from build123d import *

# Parameters (mm, degrees)
EXTRUDE_1_DEPTH     = 6.25
SKETCH_2_R          = 4
CUT_EXTRUDE_1_DEPTH = 20
SKETCH_3_R          = 4
CUT_EXTRUDE_2_DEPTH = 62.216827752
SKETCH_4_W          = 7
SKETCH_4_H          = 36
CUT_EXTRUDE_3_DEPTH = 62.216827752


with BuildPart() as part:
    # Эскиз1 → Бобышка-Вытянуть1 (new, symmetric)
    with BuildSketch(Plane(origin=(0, 0, 0), x_dir=(0, 0, -1), z_dir=(1, 0, 0))):
        Polygon((0, 49), (0, -49), (-12, -49), (-34.5, -43), (-34.5, 43), (-12, 49), align=None)
    extrude(amount=EXTRUDE_1_DEPTH, both=True)

    # Эскиз2 → Вырез-Вытянуть1 (cut)
    with BuildSketch(Plane.XY.offset(34.5)):
        with Locations((0, -5)):
            Circle(SKETCH_2_R)
        with Locations((0, -15)):
            Circle(SKETCH_2_R)
        with Locations((0, -25)):
            Circle(SKETCH_2_R)
        with Locations(Location((0, 25, 0), (0, 0, 180))):
            Circle(SKETCH_2_R)
        with Locations(Location((0, 15, 0), (0, 0, 180))):
            Circle(SKETCH_2_R)
        with Locations(Location((0, 5, 0), (0, 0, 180))):
            Circle(SKETCH_2_R)
        with Locations((0, -35)):
            Circle(SKETCH_2_R)
        with Locations(Location((0, 35, 0), (0, 0, 180))):
            Circle(SKETCH_2_R)
    extrude(amount=-CUT_EXTRUDE_1_DEPTH, mode=Mode.SUBTRACT)

    # Эскиз3 → Вырез-Вытянуть2 (cut, through all)
    with BuildSketch(Plane(origin=(6.25, 0, 0), x_dir=(0, 0, -1), z_dir=(1, 0, 0))):
        with Locations((-24.5, -35)):
            Circle(SKETCH_3_R)
        with Locations((-24.5, -25)):
            Circle(SKETCH_3_R)
        with Locations((-24.5, -15)):
            Circle(SKETCH_3_R)
        with Locations((-24.5, -5)):
            Circle(SKETCH_3_R)
        with Locations((-24.5, 5)):
            Circle(SKETCH_3_R)
        with Locations((-24.5, 15)):
            Circle(SKETCH_3_R)
        with Locations((-24.5, 25)):
            Circle(SKETCH_3_R)
        with Locations((-24.5, 35)):
            Circle(SKETCH_3_R)
    extrude(amount=-CUT_EXTRUDE_2_DEPTH, mode=Mode.SUBTRACT)

    # Эскиз4 → Вырез-Вытянуть3 (cut, through all)
    with BuildSketch(Plane.ZY.offset(6.25)):
        with Locations((3.5, 0)):
            Rectangle(SKETCH_4_W, SKETCH_4_H)
    extrude(amount=-CUT_EXTRUDE_3_DEPTH, mode=Mode.SUBTRACT)


solid = part.part
Design review of the part built by this model. Coordinates are the model's own, in mm. A direction names the side the tool comes from. Give positions to 0.01 mm unless a question says otherwise; leave off trailing zeros. Loops run counter-clockwise (first coordinate to the right, second up) from the corner with the lowest first, then second, coordinate; pieces in that order, holes last. Notation, with made-up numbers: M 62.5,63 L 90.5,63 A8 cw 90.5,70 Z; hole C 43,48 d5. An arc over 180 degrees is marked long. One line per question, with ' | ' between items. Start each with the question number.
1. To check wall thickness, follow L1, parallel to X at y = -25, z = 19.25; L2, parallel to Y at x = 2.5, z = 6; L3, parallel to Z at x = -4.25, y = 15. State the ranges of each line that lie inside material, in increasing order.
2. The part is to be moulded in two halves that separate along Z. For faces 1 (the face through (0, -49, 6)), 2 (the face through (-4.47, -1.034, 25.021)), 3 (the face through (0, -33, 0)), say which applies: released by +Z, released by -Z, zero draft, split by the parting line, or undercut.
3. Add section B-B (z = 18.5). Give the number of separate pieces and of enclosed holes in the cut face, plus the area to 3 significant figures.
4. Add section A-A (y = -35). Write out the cut boundary in (x, z), plus the area to 3 significant figures.
5. Add section C-C (y = -5). Write out the cut boundary in (x, z), plus the area to 3 significant figures.
6. Insertion check: P1, Ø5, axis at x = 3.5, z = 30, coming from the +Y side; P2, Ø4, axis at x = -0.5, y = 25.5, coming from the +Z side; P3, Ø4, axis at x = 0, y = -1, coming from the -Z side; P4, Ø5, axis at y = 5, z = 24.5, coming from the -X side. Each pin has a flat end and moves straight along its axis. Give the tip position at first contact, or say it passes through.
7. For faces 4 (the face through (-2.15, 31.627, 30.681)), 5 (the face through (0, 0, 7)), 6 (the face through (0.088, 45.958, 23.408)), list the 3-axis set-ups (+Z, -Z, +X, -X, +Y, -Y) from which the entire face can be reached by the end or side of a thin tool; tool diameter is ignored.
Worked out:
1) L1: x = -6.25 to -4, 4 to 6.25 | L2: y = -49 to -18, 18 to 49 | L3: z = 7 to 20.5, 28.5 to 34.5
2) face 1: zero draft | face 2: undercut | face 3: released by -Z
3) separate pieces: 1 | enclosed holes: 8 | area: 780 mm²
4) outline: M -6.25,0 L 6.25,0 L 6.25,20.5 L 4,20.5 L 4,14.5 L -4,14.5 L -4,20.5 L -6.25,20.5 Z; M -6.25,28.5 L -4,28.5 L -4,34.5 L -6.25,34.5 Z; M 4,28.5 L 6.25,28.5 L 6.25,34.5 L 4,34.5 Z | area: 235 mm²
5) outline: M -6.25,7 L 6.25,7 L 6.25,20.5 L 4,20.5 L 4,14.5 L -4,14.5 L -4,20.5 L -6.25,20.5 Z; M -6.25,28.5 L -4,28.5 L -4,34.5 L -6.25,34.5 Z; M 4,28.5 L 6.25,28.5 L 6.25,34.5 L 4,34.5 Z | area: 148 mm²
6) P1: stops at y = 44.87 | P2: stops at z = 14.5 | P3: stops at z = 7 | P4: passes through
7) face 4: +Z | face 5: -Z, +X, -X | face 6: +Z, +X, -X, +Y
